Verification items for the finished model (mm, model axes). A direction names the side the tool comes from. Coordinates: 2 decimals unless noted, no trailing zeros. Order: outer loops, then holes, each group sorted by start corner. A loop starts at its lowest first (then second) coordinate and runs counter-clockwise, first axis right, second up. Notation, with made-up numbers: M 37.25,54 L 92.25,54 A23 cw 92.25,75 Z; hole C 39.25,61 d9. An arc over 180 degrees is marked long. Return JSON: item names as keys, results as strings. Group by question number.
1. Set-up check for faces 4 (the flat face through (-6, 6, 6)), 5 (the flat face through (0, 31, 0)): record each of +Z, -Z, +X, -X, +Y, -Y from which the full face is reachable in a straight line by a thin tool's end or side.
2. Gauge pin test, flat ends, axial feed: pin 1 (10 mm diameter, centred on x = 15.5, y = 11, fed in from -Z); pin 2 (1.5 mm diameter, centred on x = 4, y = 12.5, fed in from +Z); pin 3 (1.5 mm diameter, centred on x = -10.5, z = 2, fed in from -Y). Record the tip position at first contact, or that the pin passes through.
3. Material ranges on line 1 along X through (y, z) = (7.75, 0); line 2 along Y through (x, z) = (-13.5, -7.5); line 3 along Y through (x, z) = (12, -19.5), recorded low to high.
4. Section check D-D, the plane y = 17. Record the cut outline in (x, z), plus the area to 3 significant figures.
5. Section check B-B, the plane z = 0. Record the cut outline in (x, y).
6. Section check A-A, the plane y = 10. Record the cut outline in (x, z), plus the area to 3 significant figures.
7. Section check C-C, the plane x = 0. Record the cut outline in (y, z), plus the area to 3 significant figures.
8. Mould release check, pull along Z, two halves, no side actions. Record for faces 1 (the flat face through (-3.4, 0, -0.1)), 2 (the flat face through (0, 15, 0)), 3 (the cylindrical face through (25.865, 12.162, 10.724)): +Z half, -Z half, draft (parallel to the pull), parting line (faces both ways), or undercut.
```python
from build123d import *

# Parameters (mm, degrees)
POCKET_DEPTH = 15


with BuildPart() as part:
    # Sketch → Revolution (revolve)
    with BuildSketch(Plane.XY):
        with BuildLine():
            Line((15.5, 31), (0, 31))
            Line((0, 31), (0, 0))
            Line((0, 0), (8, 0))
            Line((8, 0), (8, 6))
            Line((8, 6), (28, 6))
            Line((28, 18.5), (28, 6))
            ThreePointArc((28, 18.5), (25.815026, 25.56047), (20.023961, 30.15263))
            Line((20.5, 31), (20.023961, 30.15263))
            Line((15.5, 31), (20.5, 31))
        make_face()
    revolve(axis=Axis((0, 0, 0), (0, 1, 0)))

    # Sketch001 → Pocket (cut)
    with BuildSketch(Plane.XZ):
        with BuildLine():
            Line((-1.849324, 2.55), (1.849324, 2.55))
            ThreePointArc((-1.849324, 2.55), (0, -3.15), (1.849324, 2.55))
        make_face()
    extrude(amount=-POCKET_DEPTH, mode=Mode.SUBTRACT)


solid = part.part
```
Answers follow:
{
 "1": {"face 4": "-Y", "face 5": "+Z, -Z, +X, -X, +Y"},
 "2": {"pin 1": "z = -25.96", "pin 2": "z = 27.81", "pin 3": "y = 6"},
 "3": {"line 1": "-28 to -3.15, 3.15 to 28", "line 2": "6 to 31", "line 3": "6 to 28.58"},
 "4": {"outline": "C 0,0 d56", "area": "2,460 mm^2"},
 "5": {"outline": "M -28,6 L -8,6 L -8,0 L -3.15,0 L -3.15,15 L 3.15,15 L 3.15,0 L 8,0 L 8,6 L 28,6 L 28,18.5 A12.5 ccw 20.02,30.15 L 20.5,31 L -20.5,31 L -20.02,30.15 A12.5 ccw -28,18.5 Z"},
 "6": {"outline": "C 0,0 d56; hole M -1.85,2.55 A3.15 ccw long 1.85,2.55 Z", "area": "2,430 mm^2"},
 "7": {"outline": "M 0,-8 L 6,-8 L 6,-28 L 18.5,-28 A12.5 ccw 30.15,-20.02 L 31,-20.5 L 31,20.5 L 30.15,20.02 A12.5 ccw 18.5,28 L 6,28 L 6,8 L 0,8 L 0,2.55 L 15,2.55 L 15,-3.15 L 0,-3.15 Z", "area": "1,350 mm^2"},
 "8": {"face 1": "draft", "face 2": "undercut", "face 3": "parting line"}
}
